Geometry: see drawing. Coordinates: mm, zero at the bounding-box minimum. Give positions to 0.01 mm unless a question says otherwise; leave off trailing zeros. Order: outer loops, then holes, each group sorted by start corner. A loop starts at its lowest first (then second) coordinate and runs counter-clockwise, first axis right, second up. Notation, with made-up numbers: (67.25, -4.5) - (93.25, -4.5) arc R20 ccw to (93.25, 29.5) - close; hole circle Ø2 at (42, 5.5). An arc over 180 degrees is marked (long way). Write item = value, one per line. Start each with the question number.
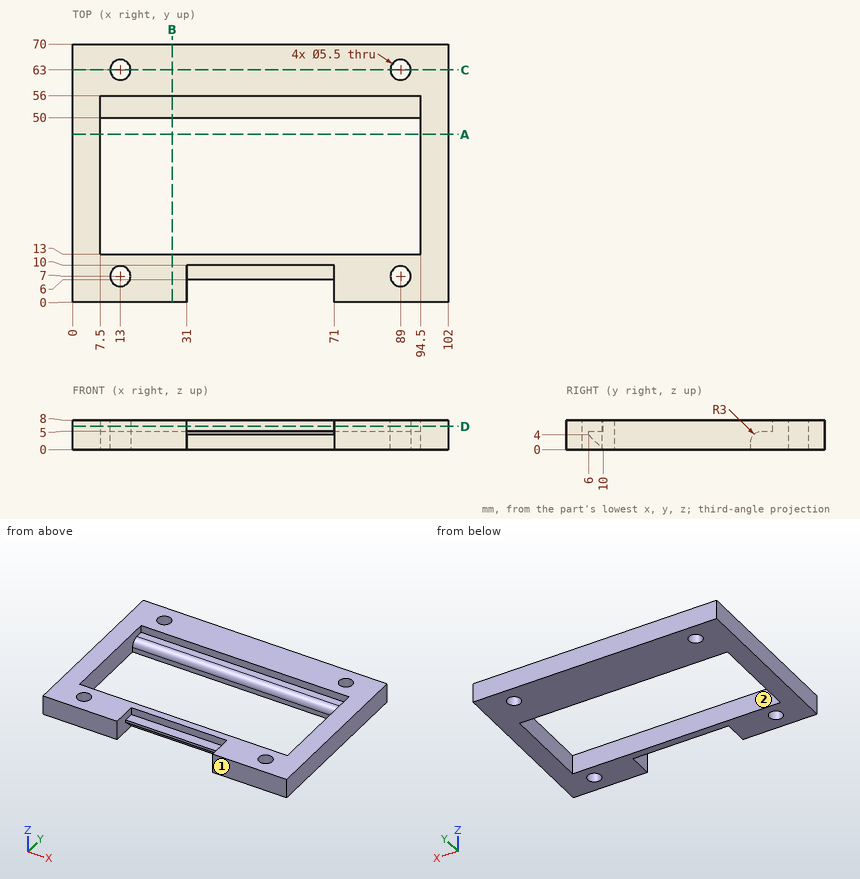
Q1. Section B-B, the plane x = 27. Return the cut outline in (y, z).
Q2. Section D-D, the plane z = 6.25. Return the cut outline in (x, y), then the cut area to 3 significant figures.
Q3. Section C-C, the plane y = 63. Return the cut outline in (x, z), then the cut area to 3 significant figures.
Q4. Contact query for flat-ended pins moving along their axis: pin 1 (4 mm diameter, centred on y = 27.5, z = 2.5, fed in from -X); pin 2 (0.8 mm diameter, centred on x = 45.5, z = 4.5, fed in from -Y); pin 3 (1.5 mm diameter, centred on x = 45.5, z = 6.5, fed in from -Y); pin 4 (2 mm diameter, centred on x = 50.5, y = 8, fed in from +Z). Output: stop coordinate, or through.
Q5. Section A-A, the plane y = 45.5. Return the cut outline in (x, z), then the cut area to 3 significant figures.
Q6. Pull-direction query (X, two-part tool) for the marked faces 1 and 2; classes: +X half, -X half, draft (parallel to the pull), parting line (faces both ways), or undercut.
Q7. Material intervals for line 1 along Y through (x, z) = (89, 5.25); line 2 along X through (y, z) = (38, 3.75); line 3 along Y through (x, z) = (72, 7.25), sorted ascending. Write a range as from..to.
The answers:
q1.outline = (0, 0) - (13, 0) - (13, 8) - (0, 8) - close; (50, 0) - (70, 0) - (70, 8) - (56, 8) - (56, 5) - (53, 5) arc R3 ccw to (50, 2) - close
q2.outline = (0, 0) - (31, 0) - (31, 10) - (71, 10) - (71, 0) - (102, 0) - (102, 70) - (0, 70) - close; hole (7.5, 13) - (94.5, 13) - (94.5, 56) - (7.5, 56) - close; hole circle Ø5.5 at (13, 7); hole circle Ø5.5 at (13, 63); hole circle Ø5.5 at (89, 7); hole circle Ø5.5 at (89, 63)
q2.area = 2,900 mm²
q3.outline = (0, 0) - (10.25, 0) - (10.25, 8) - (0, 8) - close; (15.75, 0) - (86.25, 0) - (86.25, 8) - (15.75, 8) - close; (91.75, 0) - (102, 0) - (102, 8) - (91.75, 8) - close
q3.area = 728 mm²
q4.pin_1 = 0
q4.pin_2 = 6
q4.pin_3 = 10
q4.pin_4 = 5
q5.outline = (0, 0) - (7.5, 0) - (7.5, 8) - (0, 8) - close; (94.5, 0) - (102, 0) - (102, 8) - (94.5, 8) - close
q5.area = 120 mm²
q6.face_1 = draft
q6.face_2 = undercut
q7.line_1 = 0..4.25, 9.75..13, 56..60.25, 65.75..70
q7.line_2 = 0..7.5, 94.5..102
q7.line_3 = 0..13, 56..70
